from build123d import *

# Parameters (mm, degrees)
BOSS_EXTRUDE1_DEPTH      = 11
BOSS_EXTRUDE1_DEPTH_BACK = 5
SKETCH2_R                = 3
SKETCH2_R_2              = 2
CUT_EXTRUDE1_DEPTH       = 7.3
FILLET1_R                = 1


with BuildPart() as part:
    # Sketch1 → Boss-Extrude1 (new body, two sides)
    with BuildSketch(Plane(origin=(0, 0, 0), x_dir=(1, 0, 0), z_dir=(0, 1, 0))) as boss_extrude1_sk:
        Polygon((-3.9, 0.8), (3.9, 0.8), (3.9, 0), (7.5, 0), (7.5, -3.5), (5, -5.5), (-5, -5.5), (-7.5, -3.5), (-7.5, 0), (-3.9, 0), align=None)
    extrude(amount=BOSS_EXTRUDE1_DEPTH)
    extrude(boss_extrude1_sk.sketch, amount=-BOSS_EXTRUDE1_DEPTH_BACK)

    # Sketch2 → Cut-Extrude1 (cut, through all)
    with BuildSketch(Plane(origin=(0, 0, -0.8), x_dir=(-1, 0, 0), z_dir=(0, 0, -1))):
        Circle(SKETCH2_R)
        with Locations((0, 7.5)):
            Circle(SKETCH2_R_2)
    extrude(amount=-CUT_EXTRUDE1_DEPTH, mode=Mode.SUBTRACT)

    # Fillet1
    fillet1_edges = [part.edges().sort_by_distance(p)[0] for p in [
        (7.5, 3, 0),
        (-7.5, 3, 0),
    ]]
    fillet(fillet1_edges, radius=FILLET1_R)


solid = part.part
CAD build for the part. Positions are in the model's coordinates, mm. A direction names the side the tool comes from. Round coordinates to 2 decimals unless told otherwise and drop trailing zeros. Loops run counter-clockwise (first coordinate to the right, second up) from the corner with the lowest first, then second, coordinate; pieces in that order, holes last.
(1) Cut at A-A (x = 0). Give the cut face in (y, z).
(2) Which spindle directions (+Z, -Z, +X, -X, +Y, -Y) get a long thin tool onto all of the face, cutting with end or side? Do faces 1 (the flat face through (-1, 3, -0.8)), 2 (the flat face through (5, 3, 0)), 3 (the flat face through (-5, 3, 0)). Say none if no direction does.
(3) Wall check: line 1 along Y through (x, z) = (0, 2.25); line 2 along Y through (x, z) = (-1.75, 0); line 3 along Y through (x, z) = (2.5, 0.5). Give the ranges that are in metal, low to high.
(4) Cut at C-C (z = 4.5). Give the cut face in (x, y).
(5) Cut at B-B (y = 0). Give the cut face in (x, z), plus the area to 3 significant figures.
(6) Two-plate mould, pull along X, no slides. Class faces 4 (the cylindrical face through (3, 0, 2)), 5 (the cylindrical face through (0.26, 9.483, 2.306)), 6 (the flat face through (0, 11, 2)), 7 (the cylindrical face through (-7.199, 3.112, 0.285)): +X half, -X half, draft (parallel to the pull), parting line (faces both ways), or undercut.
(7) Cut at D-D (y = 9.75). Give the cut face in (x, z).
(8) Drop flat-ended pins along their axis: pin 1 (0.9 mm diameter, centred on y = 0, z = -0.5, fed in from -X); pin 2 (5 mm diameter, centred on x = 0, y = 7.5, fed in from +Z); pin 3 (0.8 mm diameter, centred on x = -5, y = 6.5, fed in from -Z). Give the stop position or say it passes through.
Findings below:
1. outline: (-5, -0.8) - (-3, -0.8) - (-3, 5.5) - (-5, 5.5) - close; (3, -0.8) - (5.5, -0.8) - (5.5, 5.5) - (3, 5.5) - close; (9.5, -0.8) - (11, -0.8) - (11, 5.5) - (9.5, 5.5) - close
2. face 1: -Z, +X, -X, +Y, -Y
2. face 2: -Z, +X, +Y, -Y
2. face 3: -Z, -X, +Y, -Y
3. line 1: y = -5 to -3, 3 to 5.5, 9.5 to 11
3. line 2: y = -5 to -2.44, 2.44 to 6.53, 8.47 to 11
3. line 3: y = -5 to -1.66, 1.66 to 11
4. outline: (-6.25, -5) - (6.25, -5) - (6.25, 11) - (-6.25, 11) - close; hole circle Ø6 at (0, 0); hole circle Ø4 at (0, 7.5)
5. outline: (-7.5, 1) arc R1 ccw to (-6.5, 0) - (-3.9, 0) - (-3.9, -0.8) - (-3, -0.8) - (-3, 5.5) - (-5, 5.5) - (-7.5, 3.5) - close; (3, -0.8) - (3.9, -0.8) - (3.9, 0) - (6.5, 0) arc R1 ccw to (7.5, 1) - (7.5, 3.5) - (5, 5.5) - (3, 5.5) - close
5. area: 45.5 mm2
6. face 4: undercut
6. face 5: undercut
6. face 6: draft
6. face 7: -X half
7. outline: (-7.5, 1) arc R1 ccw to (-6.5, 0) - (-3.9, 0) - (-3.9, -0.8) - (3.9, -0.8) - (3.9, 0) - (6.5, 0) arc R1 ccw to (7.5, 1) - (7.5, 3.5) - (5, 5.5) - (-5, 5.5) - (-7.5, 3.5) - close
8. pin 1: stops at x = -3.9
8. pin 2: stops at z = 5.5
8. pin 3: stops at z = 0
